Answer from the drawing. Dimensions are ordinates in mm from the lowest x, y and z of the part. A direction names the side the tool comes from. Round coordinates to 2 decimals unless told otherwise and drop trailing zeros. Write each loop counter-clockwise with the first axis right and the second up, starting at its lowest first coordinate (ties: lowest second). Pieces come first, ordered by that corner, then holes. Notation, with made-up numbers: (29, 28) - (60, 28) arc R23 cw to (60, 57) - close; hole circle Ø10 at (70.5, -33.5). An arc over 180 degrees is marked (long way). One line per item, written item: value. Start each with the question number.
(1) A cutting plane is placed at C-C, the plane x = 68. Determine the outline of the cut face in (y, z), plus the area to 3 significant figures.
(2) A cutting plane is placed at D-D, the plane x = 96.5. Determine the outline of the cut face in (y, z), plus the area to 3 significant figures.
(3) For the marked faces 4 and 5, determine the directions among +Z, -Z, +X, -X, +Y, -Y from which every point of the face is accessible in a straight line to the end or side of a thin tool.
(4) A cutting plane is placed at A-A, the plane z = 51.5. Determine the outline of the cut face in (x, y).
(5) A cutting plane is placed at B-B, the plane y = 4.75. Determine the outline of the cut face in (x, z), plus the area to 3 significant figures.
(6) The mould has two halves that part along X. Classify the marked faces 1, 2 and 3: +X half, -X half, draft (parallel to the pull), parting line (faces both ways), or undercut.
(7) Find the intervals of material crossed by L1, parallel to X at y = 11, z = 62; L2, parallel to Z at x = 45, y = 9.75; L3, parallel to Z at x = 96, y = 12, in increasing order.
(8) Flat-ended cylindrical pins translate along their axes: pin 1 Ø4 at (x, y) = (122, 15.5) entering from +Z; pin 2 Ø3.5 at (y, z) = (9, 29) entering from -X; pin 3 Ø7.5 at (x, y) = (87, 10) entering from +Z. Find the tip coordinate at first contact, or state that the pin passes through.
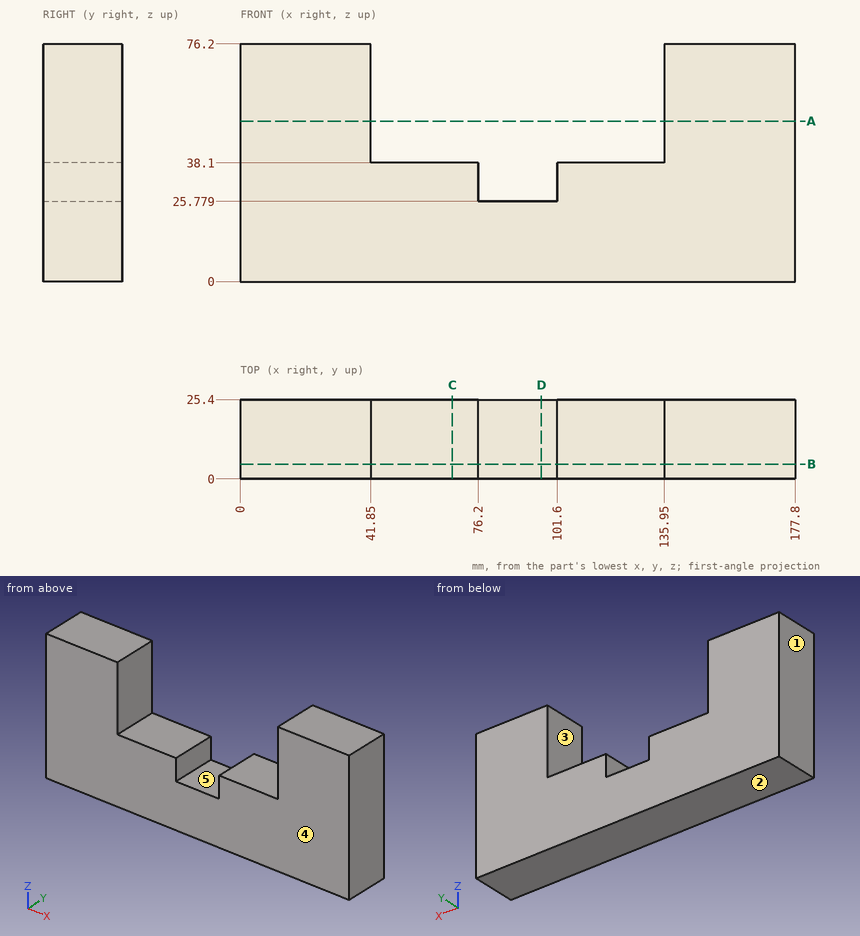
Here are the results:
1. outline: (0, 0) - (25.4, 0) - (25.4, 38.1) - (0, 38.1) - close
1. area: 968 mm²
2. outline: (0, 0) - (25.4, 0) - (25.4, 25.78) - (0, 25.78) - close
2. area: 655 mm²
3. face 4: +Z, -Z, +X, -X, -Y
3. face 5: +Z, +Y, -Y
4. outline: (0, 0) - (41.85, 0) - (41.85, 25.4) - (0, 25.4) - close; (135.95, 0) - (177.8, 0) - (177.8, 25.4) - (135.95, 25.4) - close
5. outline: (0, 0) - (177.8, 0) - (177.8, 76.2) - (135.95, 76.2) - (135.95, 38.1) - (101.6, 38.1) - (101.6, 25.78) - (76.2, 25.78) - (76.2, 38.1) - (41.85, 38.1) - (41.85, 76.2) - (0, 76.2) - close
5. area: 9,650 mm²
6. face 1: -X half
6. face 2: draft
6. face 3: undercut
7. L1: 0 to 41.85, 135.95 to 177.8
7. L2: 0 to 38.1
7. L3: 0 to 25.78
8. pin 1: z = 38.1
8. pin 2: x = 0
8. pin 3: z = 25.78
